For this review, take the finished solid that the model builds, in its own axes (mm). A direction names the side the tool comes from. Round coordinates to 2 decimals unless told otherwise and drop trailing zeros. Loops run counter-clockwise (first coordinate to the right, second up) from the corner with the lowest first, then second, coordinate; pieces in that order, holes last.
```python
from build123d import *

# Parameters (mm, degrees)
F1_DEPTH = 19.05
F2_W     = 44.45
F2_H     = 19.05
F3_DEPTH = 63.5
F5_DEPTH = 19.05


with BuildPart() as f1:
    # F0 (on Right) → F1 (new body)
    with BuildSketch(Plane.YZ):
        Polygon((-63.5, 0), (0, 0), (0, 44.45), (-19.05, 44.45), (-63.5, 12.7), align=None)
    extrude(amount=F1_DEPTH)

    # F2 (on face) → F3 (join)
    with BuildSketch(Plane(origin=(0, 0, 0), x_dir=(0, -1, 0), z_dir=(-1, 0, 0))):
        with Locations((22.225, 9.525)):
            Rectangle(F2_W, F2_H)
    extrude(amount=F3_DEPTH)

    # F4 (on face) → F5 (join)
    with BuildSketch(Plane(origin=(-63.5, 0, 0), x_dir=(0, -1, 0), z_dir=(-1, 0, 0))):
        Polygon((0, 44.214059), (0, 0), (63.867629, 0), (63.867629, 12.631163), (19.30066, 44.214059), align=None)
    extrude(amount=F5_DEPTH)


solid = f1.part
```
(1) Add section A-A (z = 41). Give the boundary of the cut face in (x, y).
(2) The part is to be moulded in two halves that separate along Z. For faces 1 (the flat face through (-31, -24, 0)), 2 (the flat face through (9.39, -40.96, 28.8)), 3 (the flat face through (-63.5, -31, 22)), say which applies: pulls with the +Z half, pulls with the -Z half, needs draft (parallel to the pull), parting line crosses it, or undercut.
(3) For faces 4 (the flat face through (-73, -10, 44.214)), 5 (the flat face through (-31, -44.45, 9)), 6 (the flat face through (0, -32, 23)), list the 3-axis set-ups (+Z, -Z, +X, -X, +Y, -Y) from which the entire face can be reached by the end or side of a thin tool; tool diameter is ignored.
(4) Add section C-C (z = 4). Give the boundary of the cut face in (x, y), plus the area to 3 significant figures.
(5) Add section B-B (y = -53.5). Give the boundary of the cut face in (x, z).
(6) Insertion check: pin 1 Ø5.5 at (x, y) = (-76, -6.5) entering from +Z; pin 2 Ø1.5 at (y, z) = (-42.5, 31) entering from -X; pin 3 Ø1.5 at (x, y) = (-18.5, -29) entering from +Z; pin 4 Ø10 at (x, z) = (6, 4) entering from -Y. Each pin has a flat end and moves straight along its axis. Give the tip position at first contact, or say it passes through.
(7) For L1, parallel to X at y = -13, z = 31; L2, parallel to Y at x = -15.5, z = 18.5; L3, parallel to Z at x = -60.5, y = -10, list the stretches that pass through material, from the lowest coordinate up.
(8) Add section D-D (y = -15.5). Give the boundary of the cut face in (x, z).
Outcome:
1. outline: (-82.55, -23.84) - (-63.5, -23.84) - (-63.5, 0) - (-82.55, 0) - close; (0, -23.88) - (19.05, -23.88) - (19.05, 0) - (0, 0) - close
2. face 1: pulls with the -Z half
2. face 2: pulls with the +Z half
2. face 3: needs draft
3. face 4: +Z, -X, +Y, -Y
3. face 5: +Z, -Z, -Y
3. face 6: +Z, -Y
4. outline: (-82.55, -63.87) - (-63.5, -63.87) - (-63.5, -44.45) - (0, -44.45) - (0, -63.5) - (19.05, -63.5) - (19.05, 0) - (-82.55, 0) - close
4. area: 5,250 mm2
5. outline: (-82.55, 0) - (-63.5, 0) - (-63.5, 19.98) - (-82.55, 19.98) - close; (0, 0) - (19.05, 0) - (19.05, 19.84) - (0, 19.84) - close
6. pin 1: stops at z = 44.21
6. pin 2: passes through
6. pin 3: stops at z = 19.05
6. pin 4: stops at y = -63.5
7. L1: x = -82.55 to -63.5, 0 to 19.05
7. L2: y = -44.45 to 0
7. L3: z = 0 to 19.05
8. outline: (-82.55, 0) - (19.05, 0) - (19.05, 44.45) - (0, 44.45) - (0, 19.05) - (-63.5, 19.05) - (-63.5, 44.21) - (-82.55, 44.21) - close
